Can you work these out from the model? Positions are in its coordinate system, mm. Face numbers are marked on the shaded views. A direction names the side the tool comes from. Give positions to 0.01 mm unless a question says otherwise; leave off trailing zeros. Order: outer loops, then holes, each group sorted by start corner. A loop starts at its lowest first (then second) coordinate and runs counter-clockwise, first axis right, second up. Notation, with made-up numbers: (-16.5, 54) -> (-9.5, 54) arc R20 cw to (-9.5, 68) -> close; hole circle Ø6 at (-34.5, 65). An arc over 180 degrees is marked (long way). Answer as a JSON object with one key per item and string values.
```python
from build123d import *

# Parameters (mm, degrees)
F0_W     = 62.23
F0_H     = 20.32
F1_DEPTH = 39.37
F2_T     = -2.54
F3_W     = 6.35
F3_H     = 3.81
F3_W_2   = 7.62
F3_H_2   = 11.43
F4_DEPTH = 25.4


with BuildPart() as f1:
    # F0 (on Front) → F1 (new body, symmetric)
    with BuildSketch(Plane.XZ):
        with Locations((-0.471618, 0)):
            Rectangle(F0_W, F0_H)
    extrude(amount=F1_DEPTH, both=True)

    # F2
    f2_openings = [f1.faces().sort_by_distance(p)[0] for p in [
        (-0.471618, 0, 10.16),
    ]]
    offset(amount=F2_T, openings=f2_openings)

    # F3 (on face) → F4 (cut)
    with BuildSketch(Plane.XZ.offset(39.37)):
        with Locations((-16.981618, -3.81)):
            Rectangle(F3_W, F3_H)
        with Locations((20.483382, 0)):
            Rectangle(F3_W_2, F3_H_2)
    extrude(amount=-F4_DEPTH, mode=Mode.SUBTRACT)


solid = f1.part
```
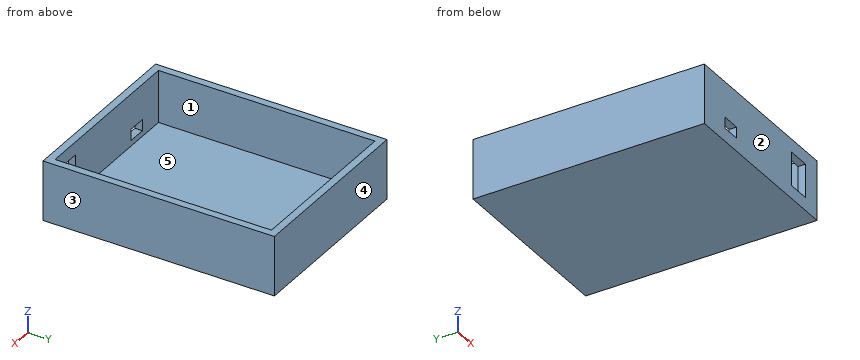
1. Will this pin go through, and if not, where does the flat tip stop? pin 1 Ø1.5 at (x, y) = (-5, -26) entering from +Z.
Worked answers:
{"pin 1": "z = -7.62"}
2. If we section it at D-D on x = -28: Please give me the cut outline in (y, z), then the cut area to 3 significant figures.
Worked answers:
{"outline": "(-39.37, -10.16) -> (39.37, -10.16) -> (39.37, 10.16) -> (36.83, 10.16) -> (36.83, -7.62) -> (-36.83, -7.62) -> (-36.83, 10.16) -> (-39.37, 10.16) -> close", "area": "290 mm²"}
3. If we section it at C-C on y = 12.5: Please give me the cut outline in (x, z).
Worked answers:
{"outline": "(-31.59, -10.16) -> (30.64, -10.16) -> (30.64, 10.16) -> (28.1, 10.16) -> (28.1, -7.62) -> (-29.05, -7.62) -> (-29.05, 10.16) -> (-31.59, 10.16) -> close"}
4. If we section it at A-A on x = -18: Please give me the cut outline in (y, z) (3 decimals).
Worked answers:
{"outline": "(-39.37, -10.16) -> (39.37, -10.16) -> (39.37, 10.16) -> (36.83, 10.16) -> (36.83, -7.62) -> (-36.83, -7.62) -> (-36.83, -5.715) -> (-39.37, -5.715) -> close; (-39.37, -1.905) -> (-36.83, -1.905) -> (-36.83, 10.16) -> (-39.37, 10.16) -> close"}
5. For the marked faces 4 and 5, which set-ups out of +Z, -Z, +X, -X, +Y, -Y let a thin tool reach every point of the face, with its end or its side?
Worked answers:
{"face 4": "+Z, -Z, +X, -X, +Y", "face 5": "+Z"}
6. Please list where these lines run through material, in increasing order: L1, parallel to X at y = -29.5, z = 5; L2, parallel to Y at x = 14, z = -1.25; L3, parallel to Z at x = 10, y = 21.
Worked answers:
{"L1": "-31.59 to -29.05, 28.1 to 30.64", "L2": "-39.37 to -36.83, 36.83 to 39.37", "L3": "-10.16 to -7.62"}
7. If we mould it in two halves opening along X, with no side actions, what happens to the marked faces 1, 2 and 3? For each: +X half, -X half, draft (parallel to the pull), parting line (faces both ways), or undercut.
Worked answers:
{"face 1": "undercut", "face 2": "draft", "face 3": "+X half"}
8. If we section it at B-B on z = 7: Please give me the cut outline in (x, y), then the cut area to 3 significant figures.
Worked answers:
{"outline": "(-31.59, -39.37) -> (30.64, -39.37) -> (30.64, 39.37) -> (-31.59, 39.37) -> close; hole (-29.05, -36.83) -> (28.1, -36.83) -> (28.1, 36.83) -> (-29.05, 36.83) -> close", "area": "690 mm²"}
